from build123d import *

# Parameters (mm, degrees)
SK_PLATE_W              = 40
SK_PLATE_H              = 40
EX_PLATE_DEPTH          = 3
SK_PLATEHOLES_4X_R      = 2.25
CUT_PLATEHOLES_4X_DEPTH = 3
SK_SWIVEL_R             = 15
EX_SWIVEL_DEPTH         = 12
SK_FORK_W               = 26
SK_FORK_H               = 26
EX_FORK_DEPTH           = 20
SK_WHEEL_R              = 25
EX_WHEEL_DEPTH          = 20


with BuildPart() as part:
    # SK_Plate → EX_Plate (new body)
    with BuildSketch(Plane(origin=(0, 0, 0), x_dir=(1, 0, 0), z_dir=(0, 1, 0))):
        Rectangle(SK_PLATE_W, SK_PLATE_H)
    extrude(amount=-EX_PLATE_DEPTH)

    # SK_PlateHoles_4x → CUT_PlateHoles_4x (cut)
    with BuildSketch(Plane(origin=(0, 0, 0), x_dir=(1, 0, 0), z_dir=(0, 1, 0))):
        with Locations(Location((15, -15, 0), (0, 0, 270))):
            Circle(SK_PLATEHOLES_4X_R)
        with Locations(Location((-15, -15, 0), (0, 0, 270))):
            Circle(SK_PLATEHOLES_4X_R)
        with Locations(Location((15, 15, 0), (0, 0, 270))):
            Circle(SK_PLATEHOLES_4X_R)
        with Locations(Location((-15, 15, 0), (0, 0, 270))):
            Circle(SK_PLATEHOLES_4X_R)
    extrude(amount=-CUT_PLATEHOLES_4X_DEPTH, mode=Mode.SUBTRACT)

    # SK_Swivel → EX_Swivel (add)
    with BuildSketch(Plane(origin=(0, -3, 0), x_dir=(1, 0, 0), z_dir=(0, 1, 0))):
        with Locations(Location((0, 0, 0), (0, 0, 270))):
            Circle(SK_SWIVEL_R)
    extrude(amount=-EX_SWIVEL_DEPTH)

    # SK_Fork → EX_Fork (add)
    with BuildSketch(Plane(origin=(0, -15, 0), x_dir=(1, 0, 0), z_dir=(0, 1, 0))):
        with Locations((0, 9)):
            Rectangle(SK_FORK_W, SK_FORK_H)
    extrude(amount=-EX_FORK_DEPTH)

    # SK_Wheel → EX_Wheel (add)
    with BuildSketch(Plane(origin=(-10, 0, 0), x_dir=(0, 0, -1), z_dir=(1, 0, 0))):
        with Locations((10, -43)):
            Circle(SK_WHEEL_R)
    extrude(amount=EX_WHEEL_DEPTH)


solid = part.part
Work out the finished part from the listing and answer in its coordinate system (mm). A direction names the side the tool comes from. Round coordinates to 2 decimals unless told otherwise and drop trailing zeros. Loops run counter-clockwise (first coordinate to the right, second up) from the corner with the lowest first, then second, coordinate; pieces in that order, holes last. Notation, with made-up numbers: (61.5, -20) - (81.5, -20) arc R22 ccw to (81.5, -6) - close; hole circle Ø3 at (-39, 62). An arc over 180 degrees is marked (long way). Use one line per item in the form item = value. Start each with the question number.
(1) Find section D-D on z = 5. Determine the outline of the cut face in (x, y), and give its area (3 significant figures).
(2) Consider line 1 (X direction, y = -1.1, z = 15); line 2 (X direction, y = -24, z = 2.5); line 3 (X direction, y = -33, z = -29). Determine where each line is inside the solid, lowest interval first.
(3) Find section A-A on z = 10.5. Determine the outline of the cut face in (x, y), and give its area (3 significant figures).
(4) Which of the six approach directions +Z, -Z, +X, -X, +Y, -Y give full straight-line access (tool end or side, diameter ignored) to faces 1 (the face through (9, -3, 13)), 2 (the face through (0, -20, -22)), 3 (the face through (0, -20, 4)), 4 (the face through (13, -25, -9)), 5 (the face through (0, -1, -20))?
(5) Flat-ended cylindrical pins translate along their axes: P1, Ø6, axis at x = -1.5, y = -26, coming from the +Z side; P2, Ø12, axis at y = -32, z = -19, coming from the -X side; P3, Ø3, axis at x = -3, y = -19.5, coming from the -Z side; P4, Ø3.5, axis at x = -15, z = -15, coming from the +Y side. Find the tip coordinate at first contact, or state that the pin passes through.
(6) Find section C-C on y = -14. Determine the outline of the cut face in (x, z).
(7) Determine the mould class of faces 6 (the face through (13.004, -1.479, -13.962)), 7 (the face through (0, -15, 6)), 8 (the face through (11, -35, -9)), 9 (the face through (0, 0, 0)) for opening direction Y: +Y half, -Y half, draft (parallel to the pull), parting line (faces both ways), or undercut.
(8) Find section B-B on x = 0. Determine the outline of the cut face in (y, z), and give its area (3 significant figures).
Answer list:
q1.outline = (-20, -3) - (-14.14, -3) - (-14.14, -15) - (14.14, -15) - (14.14, -3) - (20, -3) - (20, 0) - (-20, 0) - close; (-10, -63) - (10, -63) - (10, -23) - (-10, -23) - close
q1.area = 1,260 mm^2
q2.line_1 = -20 to -17.25, -12.75 to 12.75, 17.25 to 20
q2.line_2 = -13 to 13
q2.line_3 = -10 to 10
q3.outline = (-20, -3) - (-10.71, -3) - (-10.71, -15) - (10.71, -15) - (10.71, -3) - (20, -3) - (20, 0) - (-20, 0) - close; (-10, -57.31) - (10, -57.31) - (10, -28.69) - (-10, -28.69) - close
q3.area = 949 mm^2
q4.face_1 = none
q4.face_2 = -Z, +Y
q4.face_3 = +Z
q4.face_4 = +Z, -Z, +X, -Y
q4.face_5 = -Z, +X, -X, +Y
q5.P1 = 10.71
q5.P2 = -13
q5.P3 = -22
q5.P4 = through
q6.outline = circle Ø30 at (0, 0)
q7.face_6 = draft
q7.face_7 = undercut
q7.face_8 = -Y half
q7.face_9 = +Y half
q8.outline = (-22.29, 4) arc R25 ccw (long way) to (-21.07, -22) - (-15, -22) - (-15, -15) - (-3, -15) - (-3, -20) - (0, -20) - (0, 20) - (-3, 20) - (-3, 15) - (-15, 15) - (-15, 4) - close
q8.area = 2,550 mm^2
